from build123d import *

# Parameters (mm, degrees)
F1_DEPTH = 27.4
F0_W     = 5.625
F0_H     = 10
F2_DEPTH = 12.5
F3_DEPTH = 4.9
F5_R     = 7.242641


with BuildPart() as f1:
    # F0 (on Front) → F1 (new body, symmetric)
    with BuildSketch(Plane.XZ):
        Polygon((10, 16.25), (-10, 16.25), (-10, -16.25), (10, -16.25), (10, 10.584195), align=None)
    extrude(amount=F1_DEPTH, both=True)

    # F0 (on Front) → F2 (join, symmetric)
    with BuildSketch(Plane.XZ):
        with BuildLine():
            Line((13.125, 16.25), (10, 16.25))
            Line((10, 16.25), (10, 10.584195))
            Line((10, 10.584195), (13.125, 10.584195))
            ThreePointArc((13.125, 10.584195), (21.300311, 13.83105), (25.020355, 21.802188))
            add(Edge.make_bspline(
                [(25.020355, 21.802188), (25.02761, 22.033307), (25.034428, 22.265908), (25.040805, 22.5)],
                knots=[41.280664, 41.280664, 41.280664, 41.280664, 41.566673, 41.566673, 41.566673, 41.566673], degree=3))
            Line((25.040805, 22.5), (25.040805, 47.395553))
            Line((25.040805, 47.395553), (25, 47.395553))
            Line((25, 47.395553), (25, 37.395553))
            Line((25, 37.395553), (19.375, 37.395553))
            Line((19.375, 37.395553), (19.375, 22.5))
            ThreePointArc((19.375, 22.5), (17.544417, 18.080583), (13.125, 16.25))
        make_face()
        Polygon((13.75, 47.395553), (19.375, 47.395553), (25, 47.395553), (25, 57.395553), (13.75, 57.395553), align=None)
        with Locations((16.5625, 42.395553)):
            Rectangle(F0_W, F0_H)
        with Locations((22.1875, 42.395553)):
            Rectangle(F0_W, F0_H)
    extrude(amount=F2_DEPTH, both=True)

    # F0 (on Front) → F3 (join, symmetric)
    with BuildSketch(Plane.XZ):
        with BuildLine():
            Line((13.125, 10.584195), (10, 10.584195))
            Line((10, 10.584195), (10, -16.25))
            add(Edge.make_bspline(
                [(10, -16.25), (13.830885, -14.058451), (23.973214, -11.556052), (25.020355, 21.802188)],
                knots=[0, 0, 0, 0, 41.280664, 41.280664, 41.280664, 41.280664], degree=3))
            ThreePointArc((25.020355, 21.802188), (21.300311, 13.83105), (13.125, 10.584195))
        make_face()
    extrude(amount=F3_DEPTH, both=True)

    # F0 (on Front) → F4 (revolve)
    with BuildSketch(Plane.XZ):
        Polygon((13.75, 47.395553), (19.375, 47.395553), (25, 47.395553), (25, 57.395553), (13.75, 57.395553), align=None)
    revolve(axis=Axis((19.375, 0, 57.395553), (1, 0, 0)))

    # F5
    f5_edges = [f1.edges().sort_by_distance(p)[0] for p in [
        (0, 27.4, 16.25),
        (0, 27.4, -16.25),
        (0, -27.4, 16.25),
        (0, -27.4, -16.25),
    ]]
    fillet(f5_edges, radius=F5_R)


solid = f1.part
The listing builds one solid part. Answer for the finished solid, in the listing's coordinates (mm). A direction names the side the tool comes from. Round coordinates to 2 decimals unless told otherwise and drop trailing zeros. Order: outer loops, then holes, each group sorted by start corner. A loop starts at its lowest first (then second) coordinate and runs counter-clockwise, first axis right, second up. Notation, with made-up numbers: (-15, -18) -> (24, -18) arc R13 cw to (24, -2) -> close; hole circle Ø2 at (-33, -24). An arc over 180 degrees is marked (long way). Write each question's results on one line, items separated by ' | '. Start each with the question number.
Q1. Each of these flat-tipped pins is pushed along its axis until it touches: pin 1 (1.5 mm diameter, centred on x = 6, y = -4.5, fed in from +Z); pin 2 (12 mm diameter, centred on y = 5.5, z = 29, fed in from -X) (3 decimals); pin 3 (0.9 mm diameter, centred on x = 12, y = -8.5, fed in from -Z). Where does it stop, or does it pass through?
Q2. Find section A-A (z = 31.5). Determine the outline of the cut face in (x, y) (3 decimals).
Q3. Which of the six approach directions +Z, -Z, +X, -X, +Y, -Y give full straight-line access (tool end or side, diameter ignored) to faces 1 (the flat face through (12, 9, 10.584)), 2 (the flat face through (19, 11, 57.396)), 3 (the flat face through (16, -4.9, -1)), 4 (the flat face through (21, -12.5, 34)), 5 (the flat face through (2, 0, 16.25))?
Q4. The mould has two halves that part along Z. Classify faces 6 (the flat face through (0, 0, -16.25)), 7 (the flat face through (-10, 0, 0)), 8 (the flat face through (17, 0, 37.396)): pulls with the +Z half, pulls with the -Z half, needs draft (parallel to the pull), parting line crosses it, or undercut.
Q5. Straight lines are drawn through the part: probe 1 along Z at (x, y) = (7.5, 6.5); probe 2 along Y at (x, z) = (20.5, 41); probe 3 along X at (y, z) = (-5, 9). For each, find the intervals that lie inside material, in ascending order. Write a range as from..to.
Worked answers:
1) pin 1: stops at z = 16.25 | pin 2: stops at x = 19.375 | pin 3: stops at z = 10.58
2) outline: (19.375, -12.5) -> (25.041, -12.5) -> (25.041, 12.5) -> (19.375, 12.5) -> close
3) face 1: -Z, +X, +Y | face 2: +Z, +X, -X, +Y | face 3: -Z, +X, -Y | face 4: +Z, -Z, +X, -Y | face 5: +Z, -X, +Y, -Y
4) face 6: pulls with the -Z half | face 7: needs draft | face 8: undercut
5) probe 1: z = -16.25..16.25 | probe 2: y = -12.5..12.5 | probe 3: x = -10..10
